Study the drawing (mm; zero at the part's minimum x, y, z) and answer. A direction names the side the tool comes from. Coordinates: 2 decimals unless noted, no trailing zeros. Order: outer loops, then holes, each group sorted by start corner. A loop starts at its lowest first (then second) coordinate and runs counter-clockwise, first axis right, second up.
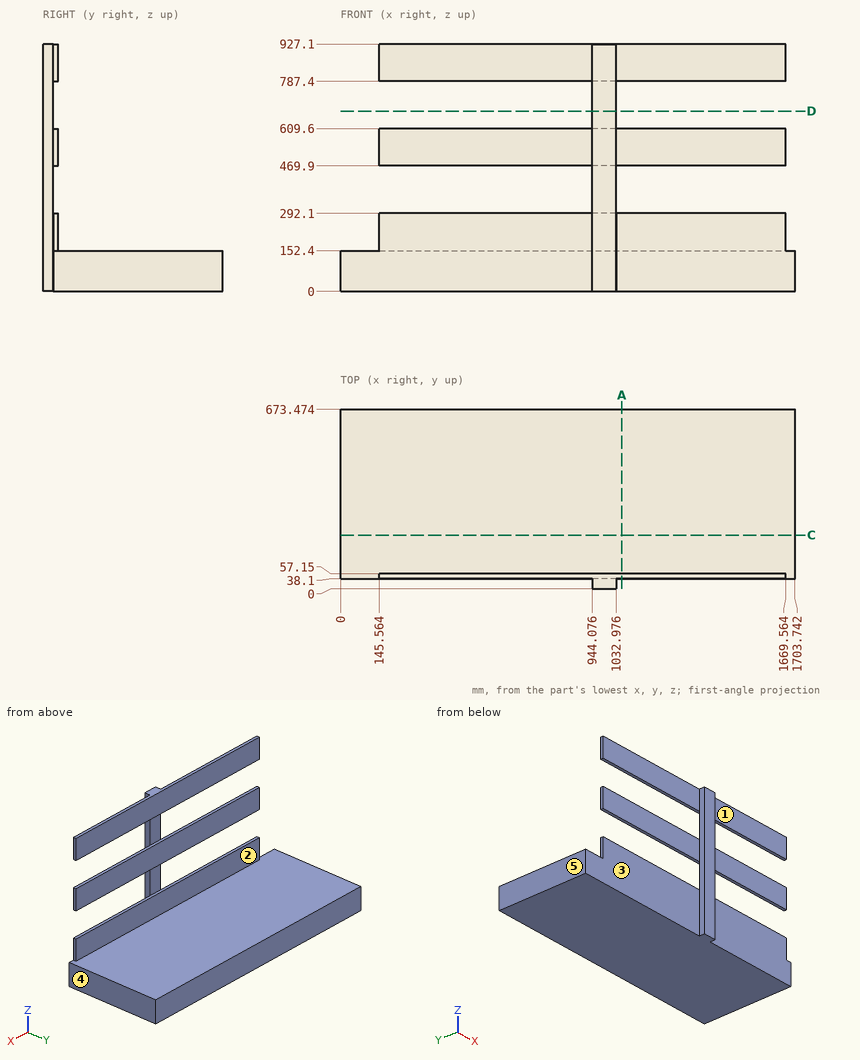
1) Straight lines are drawn through the part: line 1 (Z direction, x = 811, y = 47.5); line 2 (Z direction, x = 1275, y = 198); line 3 (Y direction, x = 967, z = 384). For each, find the intervals that lie inside material, in ascending order.
A:
line 1: z = 0 to 292.1, 469.9 to 609.6, 787.4 to 927.1
line 2: z = 0 to 152.4
line 3: y = 0 to 38.1
2) A cutting plane is placed at C-C, the plane y = 201.5. Determine the outline of the cut face in (x, z), and give its area (3 significant figures).
A:
outline: (0, 0) - (1703.74, 0) - (1703.74, 152.4) - (0, 152.4) - close
area: 260,000 mm2
3) Flat-ended cylindrical pins translate along their axes: pin 1 Ø15 at (y, z) = (46.5, 865.5) entering from +X; pin 2 Ø8 at (x, z) = (378.5, 205.5) entering from -Y; pin 3 Ø5.5 at (y, z) = (43.5, 533) entering from -X. Find the tip coordinate at first contact, or state that the pin passes through.
A:
pin 1: stops at x = 1669.56
pin 2: stops at y = 38.1
pin 3: stops at x = 145.56
4) A cutting plane is placed at D-D, the plane z = 675. Determine the outline of the cut face in (x, y), and give its area (3 significant figures).
A:
outline: (944.08, 0) - (1032.98, 0) - (1032.98, 38.1) - (944.08, 38.1) - close
area: 3,390 mm2
5) Which of the six approach directions +Z, -Z, +X, -X, +Y, -Y give full straight-line access (tool end or side, diameter ignored) to the marked faces 1, 2, 3, 4 and 5?
A:
face 1: +Z, -Z, +X, -Y
face 2: +Z, +X, -X, +Y
face 3: +Z, -Z, -X, -Y
face 4: +Z, -Z, +X, +Y, -Y
face 5: +Z, -Z, -X, +Y, -Y
6) A cutting plane is placed at A-A, the plane x = 1055. Determine the outline of the cut face in (y, z).
A:
outline: (38.1, 0) - (673.47, 0) - (673.47, 152.4) - (57.15, 152.4) - (57.15, 292.1) - (38.1, 292.1) - close; (38.1, 469.9) - (57.15, 469.9) - (57.15, 609.6) - (38.1, 609.6) - close; (38.1, 787.4) - (57.15, 787.4) - (57.15, 927.1) - (38.1, 927.1) - close
